Verification items for this drawing (mm, ordinates from the low corner). Round coordinates to 2 decimals unless told otherwise and drop trailing zeros. Loops run counter-clockwise (first coordinate to the right, second up) from the corner with the lowest first, then second, coordinate; pieces in that order, holes last. Notation, with made-up numbers: (57, 22.25) - (80, 22.25) arc R12 ccw to (80, 27.25) - close; hole circle Ø6 at (28.5, -15.5). An arc over 180 degrees is marked (long way). Answer in a Markdown table with one row per item. Add a question column.
(1) Cross-section at D-D on x = 13. Enter the section's corners in (y, z).
(2) Cross-section at A-A on x = 47.13. Enter the section's corners in (y, z), then the cut area to 3 significant figures.
(3) Thickness scan on line 1 along X through (y, z) = (12, 83.22); line 2 along Z through (x, y) = (47.13, 14.75); line 3 along X through (y, z) = (9, 93.25). Record the ranges inside material, lowest first.
(4) Cross-section at C-C on y = 21.75. Enter the section's corners in (x, z).
(5) Gauge pin test, flat ends, axial feed: pin 1 (4 mm diameter, centred on x = 47.13, z = 83.22, fed in from -Y); pin 2 (2.5 mm diameter, centred on y = 7.5, z = 101, fed in from +X); pin 3 (0.9 mm diameter, centred on x = 17, z = 98.5, fed in from +Y); pin 4 (3.5 mm diameter, centred on x = 14.5, z = 100.5, fed in from -Y). Record the tip position at first contact, or that the pin passes through.
(6) Cross-section at B-B on z = 83.22. Enter the section's corners in (x, y).
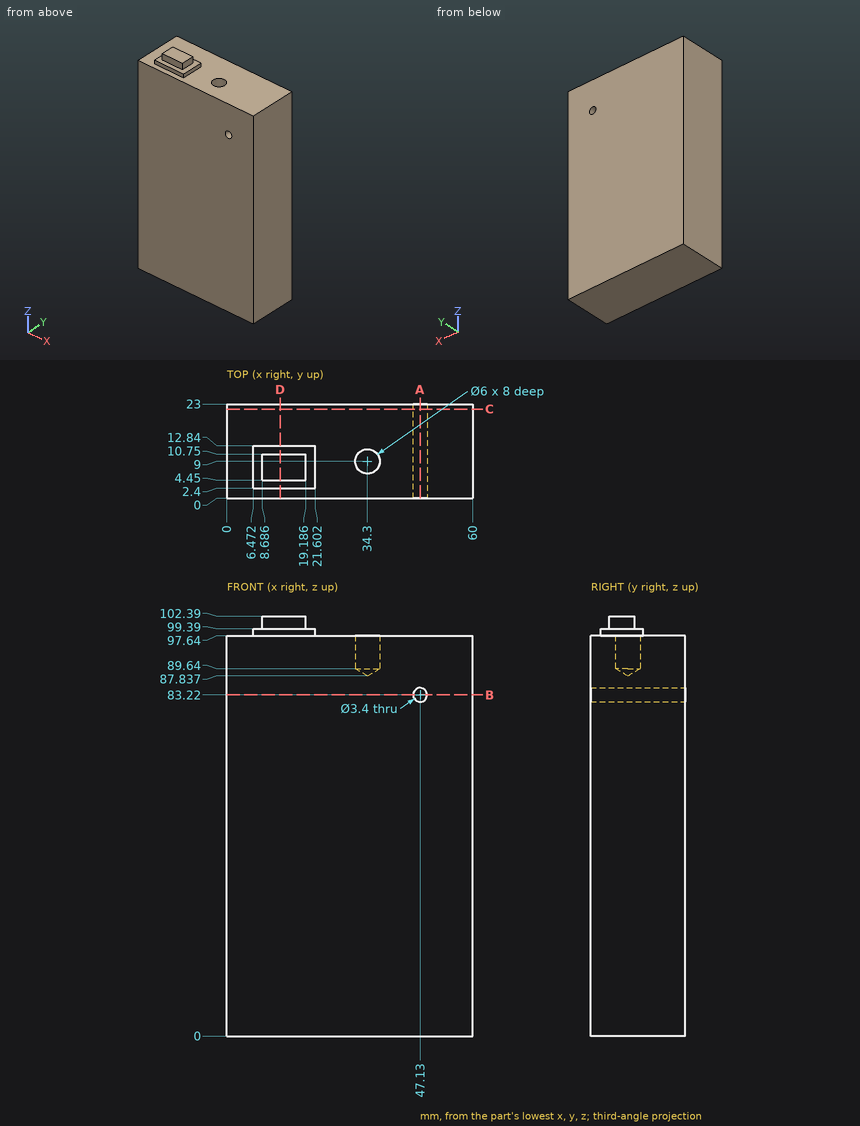
Answers:
| question | item | result |
|---|---|---|
| 1 | outline | (0, 0) - (23, 0) - (23, 97.64) - (12.84, 97.64) - (12.84, 99.39) - (10.75, 99.39) - (10.75, 102.39) - (4.45, 102.39) - (4.45, 99.39) - (2.4, 99.39) - (2.4, 97.64) - (0, 97.64) - close |
| 2 | outline | (0, 0) - (23, 0) - (23, 81.52) - (0, 81.52) - close; (0, 84.92) - (23, 84.92) - (23, 97.64) - (0, 97.64) - close |
| 2 | area | 2,170 mm^2 |
| 3 | line 1 | x = 0 to 45.43, 48.83 to 60 |
| 3 | line 2 | z = 0 to 81.52, 84.92 to 97.64 |
| 3 | line 3 | x = 0 to 31.3, 37.3 to 60 |
| 4 | outline | (0, 0) - (60, 0) - (60, 97.64) - (0, 97.64) - close; hole circle Ø3.4 at (47.13, 83.22) |
| 5 | pin 1 | stops at y = 0 |
| 5 | pin 2 | stops at x = 19.19 |
| 5 | pin 3 | stops at y = 12.84 |
| 5 | pin 4 | stops at y = 2.4 |
| 6 | outline | (0, 0) - (45.43, 0) - (45.43, 23) - (0, 23) - close; (48.83, 0) - (60, 0) - (60, 23) - (48.83, 23) - close |
